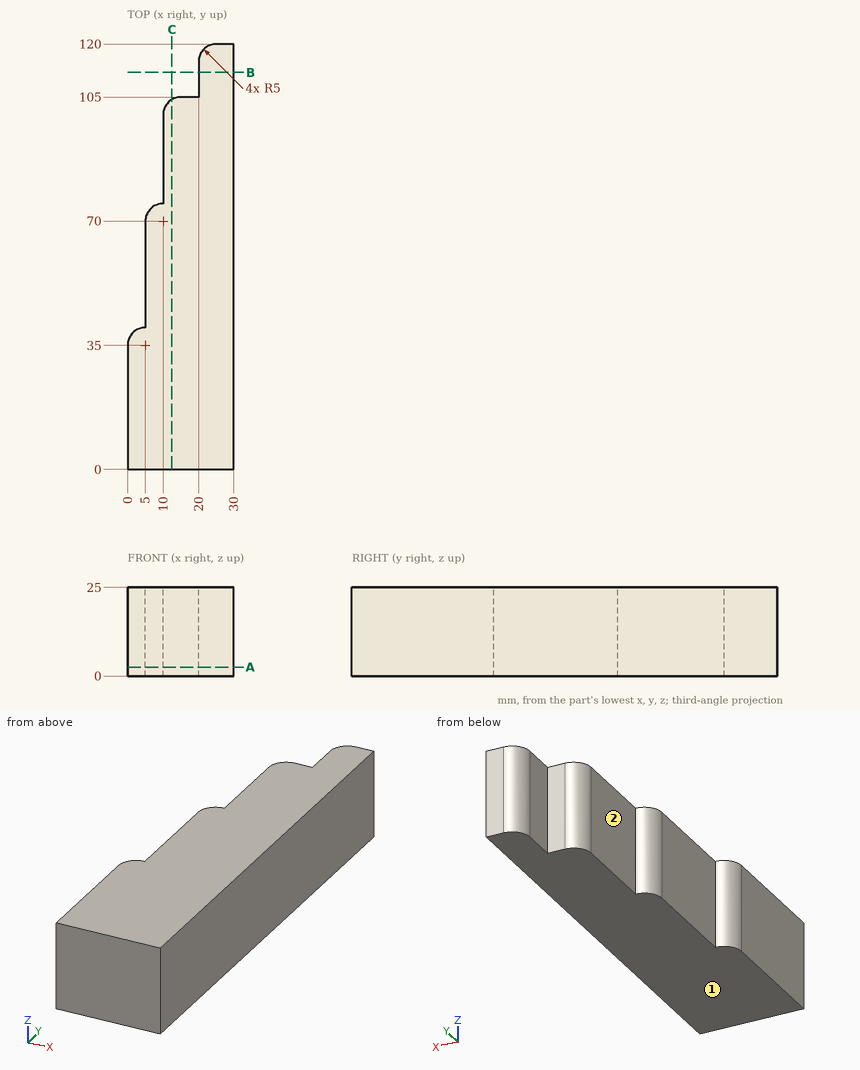
Check sheet for the drawn part. Datum: minimum x, y, z corner. Units: mm. A direction names the side the tool comes from. Round coordinates to 2 decimals unless told otherwise and drop trailing zeros. Order: outer loops, then holes, each group sorted by start corner. A loop starts at its lowest first (then second) coordinate and runs counter-clockwise, first axis right, second up. Notation, with made-up numbers: (34, -9) -> (84, -9) arc R17 ccw to (84, 2) -> close; hole circle Ø9 at (62.5, -22.75). An arc over 180 degrees is marked (long way). Put each result on its own line as item: value.
1) Depth check by flat-ended pin: pin 1 (12.5 mm diameter, centred on y = 83, z = 17.5, fed in from -X); pin 2 (6 mm diameter, centred on x = 4, z = 3, fed in from +Y); pin 3 (3 mm diameter, centred on y = 108, z = 16, fed in from -X). Enter the tip coordinate at first touch or a pass-through.
Final values:
pin 1: stops at x = 10
pin 2: stops at y = 74
pin 3: stops at x = 20
2) Section check A-A (z = 2.5). Record the cut outline in (x, y).
Final values:
outline: (0, 0) -> (30, 0) -> (30, 120) -> (25, 120) arc R5 ccw to (20, 115) -> (20, 105) -> (15, 105) arc R5 ccw to (10, 100) -> (10, 75) arc R5 ccw to (5, 70) -> (5, 40) arc R5 ccw to (0, 35) -> close
3) Material ranges on line 1 (X direction, y = 65, z = 7.5); line 2 (Y direction, x = 18.5, z = 11.25); line 3 (Y direction, x = 8.5, z = 14.5), recorded low to high.
Final values:
line 1: x = 5 to 30
line 2: y = 0 to 105
line 3: y = 0 to 74.77
4) Section check C-C (x = 12.5). Record the cut outline in (y, z), then the cut area to 3 significant figures.
Final values:
outline: (0, 0) -> (104.33, 0) -> (104.33, 25) -> (0, 25) -> close
area: 2,610 mm^2
5) Section check B-B (y = 112). Record the cut outline in (x, z), then the cut area to 3 significant figures.
Final values:
outline: (20, 0) -> (30, 0) -> (30, 25) -> (20, 25) -> close
area: 250 mm^2
6) Set-up check for the marked faces 1 and 2: record each of +Z, -Z, +X, -X, +Y, -Y from which the full face is reachable in a straight line by a thin tool's end or side.
Final values:
face 1: -Z, +X, -X, +Y, -Y
face 2: +Z, -Z, -X, +Y
